Could you check a few things on this model? Use its own coordinates, in mm. A direction names the side the tool comes from. Give positions to 0.01 mm unless a question says otherwise; leave off trailing zeros. Write each loop counter-clockwise with the first axis right and the second up, starting at its lowest first coordinate (ties: lowest second). Pieces come first, ordered by that corner, then holes. Notation, with made-up numbers: M 32.5,-0.75 L 72.5,-0.75 A33 cw 72.5,34.25 Z; hole C 32,-11 d4. An arc over 180 degrees is marked long. Answer as a JSON object with one key per item and string values. Group by question number.
```python
from build123d import *

# Parameters (mm, degrees)
SKETCH1_W           = 42.12
SKETCH1_H           = 40.42
BOSS_EXTRUDE1_DEPTH = 0.01
SKETCH2_W           = 42.12
SKETCH2_H           = 40.42
BOSS_EXTRUDE2_DEPTH = 2.92
SKETCH3_W           = 42.12
SKETCH3_H           = 3.12
BOSS_EXTRUDE3_DEPTH = 39
SKETCH4_R           = 1
CUT_EXTRUDE1_DEPTH  = 62.930807358
SKETCH5_R           = 9.087989047
CUT_EXTRUDE2_DEPTH  = 1


with BuildPart() as part:
    # Sketch1 → Boss-Extrude1 (new body)
    with BuildSketch(Plane(origin=(0, 0, 0), x_dir=(0, 0, -1), z_dir=(1, 0, 0))):
        with Locations((0, 20.21)):
            Rectangle(SKETCH1_W, SKETCH1_H)
    extrude(amount=BOSS_EXTRUDE1_DEPTH)

    # Sketch2 → Boss-Extrude2 (add)
    with BuildSketch(Plane(origin=(0.01, 0, 0), x_dir=(0, 0, -1), z_dir=(1, 0, 0))):
        with Locations((0, 20.21)):
            Rectangle(SKETCH2_W, SKETCH2_H)
    extrude(amount=BOSS_EXTRUDE2_DEPTH)

    # Sketch3 → Boss-Extrude3 (add)
    with BuildSketch(Plane(origin=(2.93, 0, 0), x_dir=(0, 0, -1), z_dir=(1, 0, 0))):
        with Locations((0, 1.56)):
            Rectangle(SKETCH3_W, SKETCH3_H)
    extrude(amount=BOSS_EXTRUDE3_DEPTH)

    # Sketch4 → Cut-Extrude1 (cut, through all)
    with BuildSketch(Plane.ZY):
        with Locations((15.42, 16.14)):
            Circle(SKETCH4_R)
        with Locations((-15.42, 16.14)):
            Circle(SKETCH4_R)
    extrude(amount=-CUT_EXTRUDE1_DEPTH, mode=Mode.SUBTRACT)

    # Sketch5 → Cut-Extrude2 (cut)
    with BuildSketch(Plane.XZ):
        with Locations(Location((25.93, 0, 0), (0, 0, 270))):
            Circle(SKETCH5_R)
    extrude(amount=-CUT_EXTRUDE2_DEPTH, mode=Mode.SUBTRACT)


solid = part.part
```
1) If we section it at A-A, the plane y = 16.14: List the corners of the cut face in (x, z) for me.
2) Please list where these lines run through material, in increasing order: line 1 along Z through (x, y) = (2, 16); line 2 along Y through (x, z) = (0.75, -15.42); line 3 along Y through (x, z) = (38.5, 6). Write a range as from..to.
3) If we section it at B-B, the plane z = -15.42: List the corners of the cut face in (x, y) for me, plus the area to 3 significant figures.
4) We'd pull the mould along X, two halves only. Please class faces 1 (the flat face through (0, 20, 0)), 2 (the flat face through (12, 2, -21.06)), 3 (the cylindrical face through (17.06, 0.49, 1.97)): released by +X, released by -X, zero draft, split by the parting line, or undercut.
5) For faces 4 (the flat face through (22, 3.12, 0)), 5 (the flat face through (41.93, 2, 0)), 6 (the flat face through (26, 1, 0)), which set-ups out of +Z, -Z, +X, -X, +Y, -Y let a thin tool reach every point of the face, with its end or its side?
6) If we section it at C-C, the plane x = 25.93: List the corners of the cut face in (y, z) for me.
7) I'm going to push flat-ended pins straight in: pin 1 (10 mm diameter, centred on x = 32, z = 9, fed in from +Y); pin 2 (1.5 mm diameter, centred on y = 21.5, z = -5.5, fed in from +X); pin 3 (16.5 mm diameter, centred on x = 25.93, z = 0, fed in from -Y). Where does each tip first touch, or does it pass through?
8) If we section it at D-D, the plane z = 0: List the corners of the cut face in (x, y) for me.
Taken from the geometry:
{
 "1": {"outline": "M 0,-21.06 L 2.93,-21.06 L 2.93,-16.42 L 0,-16.42 Z; M 0,-14.42 L 2.93,-14.42 L 2.93,14.42 L 0,14.42 Z; M 0,16.42 L 2.93,16.42 L 2.93,21.06 L 0,21.06 Z"},
 "2": {"line 1": "-21.06..-16.41, -14.43..14.43, 16.41..21.06", "line 2": "0..15.14, 17.14..40.42", "line 3": "0..3.12"},
 "3": {"outline": "M 0,0 L 41.93,0 L 41.93,3.12 L 2.93,3.12 L 2.93,15.14 L 0,15.14 Z; M 0,17.14 L 2.93,17.14 L 2.93,40.42 L 0,40.42 Z", "area": "234 mm²"},
 "4": {"face 1": "released by -X", "face 2": "zero draft", "face 3": "undercut"},
 "5": {"face 4": "+Z, -Z, +X, +Y", "face 5": "+Z, -Z, +X, +Y, -Y", "face 6": "-Y"},
 "6": {"outline": "M 0,-21.06 L 3.12,-21.06 L 3.12,21.06 L 0,21.06 L 0,9.09 L 1,9.09 L 1,-9.09 L 0,-9.09 Z"},
 "7": {"pin 1": "y = 3.12", "pin 2": "x = 2.93", "pin 3": "y = 1"},
 "8": {"outline": "M 0,0 L 16.84,0 L 16.84,1 L 35.02,1 L 35.02,0 L 41.93,0 L 41.93,3.12 L 2.93,3.12 L 2.93,40.42 L 0,40.42 Z"}
}
